For this review, use the dimensioned drawing (mm, ordinates from the lowest corner) and the shaded views. A direction names the side the tool comes from. Coordinates: 2 decimals unless noted, no trailing zeros. Write each loop counter-clockwise with the first axis right and the second up, starting at its lowest first coordinate (ties: lowest second). Pieces come first, ordered by that corner, then holes. Notation, with made-up numbers: (21, -35) - (53, -35) arc R15 ccw to (53, -11) - close; hole circle Ø8 at (58.5, 8.25). An arc over 180 degrees is marked (long way). Put each result on its own line as item: value.
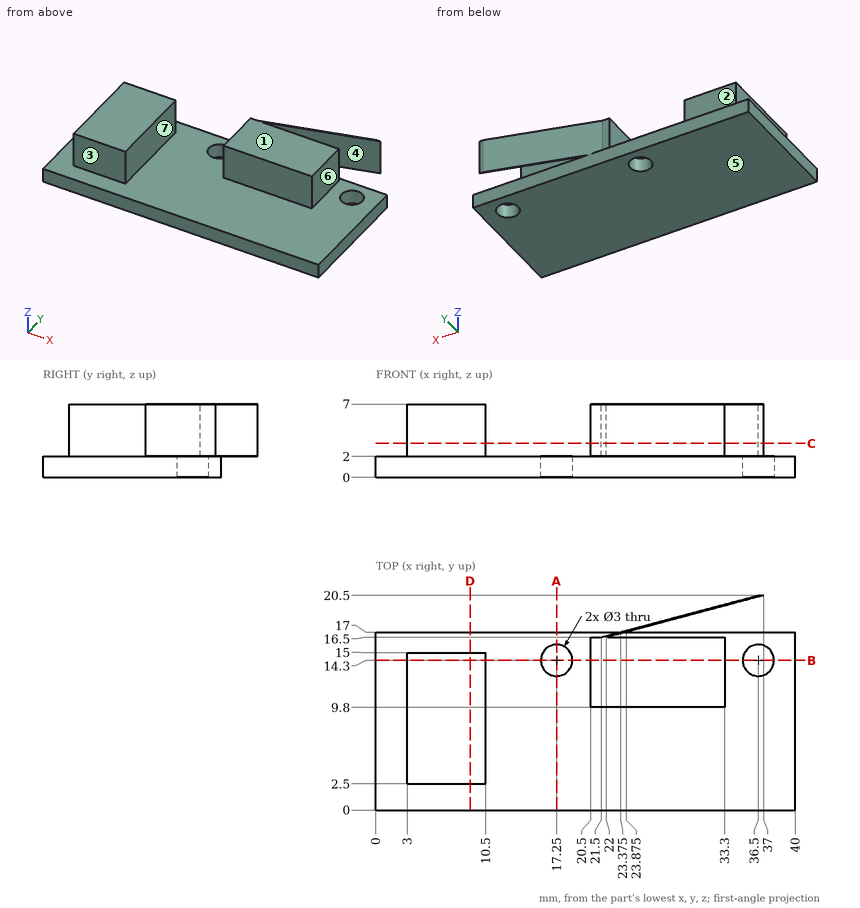
1. Consider section D-D on x = 9. State the section outline as (y, z) points.
Determined:
outline: (0, 0) - (17, 0) - (17, 2) - (15, 2) - (15, 7) - (2.5, 7) - (2.5, 2) - (0, 2) - close
2. To check wall thickness, follow probe 1 along Y at (x, z) = (36.5, 1.35); probe 2 along Z at (x, y) = (34.5, 8.75); probe 3 along X at (y, z) = (12.75, 6.5). State the ranges of each line that lie inside material, in increasing order.
Determined:
probe 1: y = 0 to 12.8, 15.8 to 17
probe 2: z = 0 to 2
probe 3: x = 3 to 10.5, 20.5 to 33.3
3. The part is to be moulded in two halves that separate along Y. For the marked faces 1, 2, 3 and 4, say which applies: +Y half, -Y half, draft (parallel to the pull), parting line (faces both ways), or undercut.
Determined:
face 1: draft
face 2: +Y half
face 3: -Y half
face 4: undercut
4. Consider section A-A on x = 17.25. State the section outline as (y, z) points.
Determined:
outline: (0, 0) - (12.8, 0) - (12.8, 2) - (0, 2) - close; (15.8, 0) - (17, 0) - (17, 2) - (15.8, 2) - close
5. Consider section B-B on y = 14.3. State the section outline as (x, z) points.
Determined:
outline: (0, 0) - (15.75, 0) - (15.75, 2) - (10.5, 2) - (10.5, 7) - (3, 7) - (3, 2) - (0, 2) - close; (18.75, 0) - (35, 0) - (35, 2) - (33.3, 2) - (33.3, 7) - (20.5, 7) - (20.5, 2) - (18.75, 2) - close; (38, 0) - (40, 0) - (40, 2) - (38, 2) - close
6. Machinability: for the marked faces 5, 6 and 7, which of the approach directions +Z, -Z, +X, -X, +Y, -Y give a long, thin tool a straight path to every point of the face, cutting with its end or side? Answer none if there is none.
Determined:
face 5: -Z, +X, -X, +Y, -Y
face 6: +Z, +X, -Y
face 7: +Z, +Y, -Y
7. Consider section C-C on z = 3.25. State the section outline as (x, y) points, plus the area to 3 significant figures.
Determined:
outline: (3, 2.5) - (10.5, 2.5) - (10.5, 15) - (3, 15) - close; (20.5, 9.8) - (33.3, 9.8) - (33.3, 16.5) - (22, 16.5) - (37, 20.5) - (36.5, 20.5) - (21.5, 16.5) - (20.5, 16.5) - close
area: 182 mm^2
8. For pin 1 Ø2.5 at (x, z) = (28, 5) entering from +Y; pin 2 Ø4 at (x, y) = (17.25, 14.3) entering from +Z; pin 3 Ø1.5 at (y, z) = (13, 4) entering from -X, all flat-tipped, find the tip position at first contact; note any pin that passes through.
Determined:
pin 1: stops at y = 18.57
pin 2: stops at z = 2
pin 3: stops at x = 3
